Here's how the part is built. I have some questions about the finished solid (model axes, mm). A direction names the side the tool comes from. Coordinates: 2 decimals unless noted, no trailing zeros. Write each loop counter-clockwise with the first axis right and the second up, starting at its lowest first coordinate (ties: lowest second). Pieces come first, ordered by that corner, then holes. Notation, with made-up numbers: M -26,-19.75 L 23,-19.75 A8 ccw 23,-8.75 Z; hole C 74,67.25 d5. An arc over 180 degrees is marked long. Use one line per item in the form item = value. Start each with the question number.
1. On a 3-axis mill with a long thin cutter (end or side, diameter ignored), from which of +Z, -Z, +X, -X, +Y, -Y can I reach the whole of each face in a straight line? I mean faces 1 (the face through (-6, -6, -255)), 2 (the face through (10, 27, -35)). Say none if no direction works.
2. I want a section at C-C, the plane y = 7.5. List the corners of the cut face in (x, z) for me.
3. Thinking about a two-plate mould opening in Y: for faces 3 (the face through (8, 30, -35)), 4 (the face through (-6, -6, 255)), 5 (the face through (-18.5, -19.7, 3.6)), 6 (the face through (10, 27, 170)), which applies, released by +Y, released by -Y, zero draft, split by the parting line, or undercut?
4. Please list where these lines run through material, in increasing order: line 1 along Y through (x, z) = (10, -209.5); line 2 along Y through (x, z) = (-2, -133); line 3 along X through (y, z) = (12, 12.5). Write a range as [from, to].
5. I want a section at D-D, the plane x = -9. List the corners of the cut face in (y, z) for me, plus the area to 3 significant figures.
6. I'm going to push flat-ended pins straight in: pin 1 Ø4 at (y, z) = (-9, -154.5) entering from +X; pin 2 Ø0.9 at (x, z) = (-1.5, 229.5) entering from +Y; pin 3 Ø0.9 at (x, y) = (12, 28.5) entering from +Z; pin 4 Ø3.5 at (y, z) = (29, 46.5) entering from -X. Where does each tip first touch, or does it pass through?
7. I want a section at A-A, the plane x = 14. List the corners of the cut face in (y, z) for me, plus the area to 3 significant figures.
8. I want a section at B-B, the plane z = 7.5. List the corners of the cut face in (x, y) for me.
from build123d import *

# Parameters (mm, degrees)
BOSS_EXTRUDE1_DEPTH = 255
SKETCH5_W           = 23
SKETCH5_H           = 20
BOSS_EXTRUDE2_DEPTH = 3
BOSS_EXTRUDE3_DEPTH = 3


with BuildPart() as part:
    # Sketch4 → Boss-Extrude1 (new, symmetric)
    with BuildSketch(Plane.XY):
        with BuildLine():
            Line((0, 0), (27, 0))
            Line((27, 0), (27, -3))
            Line((27, -3), (26.800082477, -3))
            ThreePointArc((26.800082477, -3), (-19.135504983, -19.08508544), (-3, 26.83281573))
            Line((-3, 26.83281573), (-3, 27))
            Line((-3, 27), (0, 27))
            Line((0, 27), (0, 0))
        make_face()
    extrude(amount=BOSS_EXTRUDE1_DEPTH, both=True)

    # Sketch5 → Boss-Extrude2 (add)
    with BuildSketch(Plane(origin=(0, 27, 0), x_dir=(1, 0, 0), z_dir=(0, 1, 0))):
        with Locations((8.5, -170)):
            Rectangle(SKETCH5_W, SKETCH5_H)
        with Locations((8.5, 35)):
            Rectangle(SKETCH5_W, SKETCH5_H)
    extrude(amount=BOSS_EXTRUDE2_DEPTH)

    # Sketch6 → Boss-Extrude3 (add)
    with BuildSketch(Plane(origin=(-3, 27, 180), x_dir=(0, 0, -1), z_dir=(1, 0, 0))):
        with BuildLine():
            ThreePointArc((0, 2.5), (-0.732233047, 0.732233047), (-2.5, 0))
            Line((-2.5, 0), (0, 0))
            Line((0, 0), (0, 2.5))
        make_face()
    extrude(amount=BOSS_EXTRUDE3_DEPTH)


solid = part.part
Answer list:
q1.face_1 = -Z, +X, -X, +Y, -Y
q1.face_2 = +Z, -Z, +X
q2.outline = M -25.97,-255 L 0,-255 L 0,255 L -25.97,255 Z
q3.face_3 = released by +Y
q3.face_4 = zero draft
q3.face_5 = split by the parting line
q3.face_6 = undercut
q4.line_1 = [-25.07, 0]
q4.line_2 = [-26.93, 27]
q4.line_3 = [-24.22, 0]
q5.outline = M -25.47,-255 L 25.46,-255 L 25.46,255 L -25.47,255 Z
q5.area = 26,000 mm²
q6.pin_1 = 26.04
q6.pin_2 = 27
q6.pin_3 = 180
q6.pin_4 = through
q7.outline = M -23.07,-255 L 0,-255 L 0,255 L -23.07,255 Z; M 27,-45 L 30,-45 L 30,-25 L 27,-25 Z; M 27,160 L 30,160 L 30,180 L 27,180 Z
q7.area = 11,900 mm²
q8.outline = M -3,26.83 A27 ccw long 26.8,-3 L 27,-3 L 27,0 L 0,0 L 0,27 L -3,27 Z
